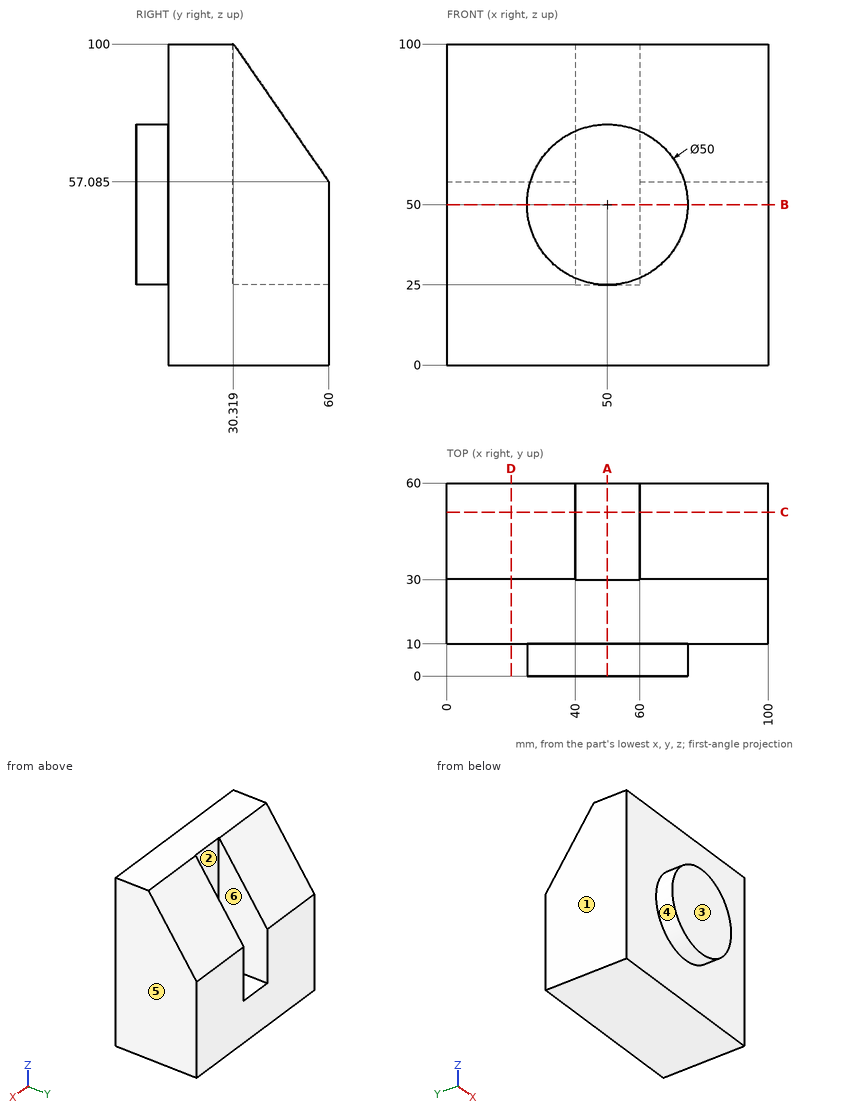
Verification items for this drawing (mm, ordinates from the low corner). A direction names the side the tool comes from. Round coordinates to 2 decimals unless told otherwise and drop trailing zeros. Order: outer loops, then holes, each group sorted by start corner. A loop starts at its lowest first (then second) coordinate and runs counter-clockwise, first axis right, second up. Notation, with made-up numbers: (-27.75, -5.5) - (14.25, -5.5) arc R15 ccw to (14.25, 16.5) - close; hole circle Ø5 at (68.5, -36.5). An arc over 180 degrees is marked (long way). Answer as CSV lines item,"result". Start each with the question number.
1) Tool access check on the marked faces 4, 5 and 6. Record the directions out of +Z, -Z, +X, -X, +Y, -Y that give a thin tool (end or side, any length) a straight path to the whole face; none if there is none.
2) Section check B-B (z = 50). Record the cut outline in (x, y).
3) Section check C-C (y = 51). Record the cut outline in (x, z), then the cut area to 3 significant figures.
4) Scan lines: probe 1 along X at (y, z) = (55.5, 53.5); probe 2 along Y at (x, z) = (49.5, 40.5); probe 3 along Y at (x, z) = (89, 41). Record each from-to range of solid material in increasing order.
5) Draft check along X on the marked faces 1, 2 and 3. Enter one of: +X half, -X half, draft (parallel to the pull), parting line (faces both ways), or undercut.
6) Depth check by flat-ended pin: pin 1 (8 mm diameter, centred on x = 58.5, y = 42, fed in from +Z) (1 decimal); pin 2 (6 mm diameter, centred on x = 64, z = 81.5, fed in from +Y); pin 3 (10 mm diameter, centred on x = 46.5, z = 44.5, fed in from +Y). Enter the tip coordinate at first touch or a pass-through.
7) Section check D-D (x = 20). Record the cut outline in (y, z) (1 decimal), then the cut area to 3 significant figures.
8) Section check A-A (x = 50). Record the cut outline in (y, z).
Determined:
1,face 4,"-Y"
1,face 5,"+Z, -Z, +X, +Y, -Y"
1,face 6,"+Z, +Y"
2,outline,"(0, 10) - (25, 10) - (25, 0) - (75, 0) - (75, 10) - (100, 10) - (100, 60) - (60, 60) - (60, 30) - (40, 30) - (40, 60) - (0, 60) - close"
3,outline,"(0, 0) - (100, 0) - (100, 70.1) - (60, 70.1) - (60, 25) - (40, 25) - (40, 70.1) - (0, 70.1) - close"
3,area,"6,110 mm^2"
4,probe 1,"0 to 40, 60 to 100"
4,probe 2,"0 to 30"
4,probe 3,"10 to 60"
5,face 1,"-X half"
5,face 2,"undercut"
5,face 3,"draft"
6,pin 1,"z = 88.5"
6,pin 2,"y = 45.19"
6,pin 3,"y = 30"
7,outline,"(10, 0) - (60, 0) - (60, 57.1) - (30.3, 100) - (10, 100) - close"
7,area,"4,360 mm^2"
8,outline,"(0, 25) - (10, 25) - (10, 0) - (60, 0) - (60, 25) - (30, 25) - (30, 100) - (10, 100) - (10, 75) - (0, 75) - close"
